```python
from build123d import *

# Parameters (mm, degrees)
BOSS_EXTRUDE1_DEPTH = 28
FILLET1_R           = 1
SWEEP1_PROFILE_R    = 0.7
LPATTERN1_COUNT     = 2
LPATTERN1_PITCH     = 2.5


with BuildPart() as part:
    # Sketch1 → Boss-Extrude1 (new body)
    with BuildSketch(Plane(origin=(0, 0, 0), x_dir=(0, 0, -1), z_dir=(1, 0, 0))):
        Polygon((0, 0), (0, 31), (2, 31), (5.7, 24), (5.7, 0), align=None)
    extrude(amount=BOSS_EXTRUDE1_DEPTH)

    # Fillet1
    fillet1_edges = [part.edges().sort_by_distance(p)[0] for p in [
        (28, 15.5, 0),
        (28, 31, -1),
        (28, 27.5, -3.85),
        (28, 12, -5.7),
        (0, 27.5, -3.85),
        (0, 31, -1),
        (0, 15.5, 0),
        (0, 0, -2.85),
        (0, 12, -5.7),
        (28, 0, -2.85),
        (14, 24, -5.7),
        (14, 31, -2),
        (14, 31, 0),
        (14, 0, 0),
        (14, 0, -5.7),
    ]]
    fillet(fillet1_edges, radius=FILLET1_R)

    # Sweep1: sweep along a path in Sketch2
    with BuildLine(Plane.XY.offset(-1.3)) as sweep1_path:
        ThreePointArc((2.353185581, 32.918653967), (1.45227767, 31.219358637), (2.297855958, 29.491864196))
    # Sweep1 profile (on start of the path) → Sweep1 (sweep)
    with BuildSketch(Plane(origin=(2.353185581, 32.918653967, -1.3), x_dir=(0.5744773116902536, -0.8185205057621582, 0), z_dir=(-0.8185205057621582, -0.5744773116902536, 0))):
        Circle(SWEEP1_PROFILE_R)
    sweep1 = sweep(path=sweep1_path.line)

    # LPattern1: Sweep1 ×2
    with Locations(*[(i * LPATTERN1_PITCH, 0, 0) for i in range(1, LPATTERN1_COUNT)]):
        add(sweep1)


solid = part.part
```
Here's how the part is built. I have some questions about the finished solid (model axes, mm). Give positions to 0.01 mm unless a question says otherwise; leave off trailing zeros. Loops run counter-clockwise (first coordinate to the right, second up) from the corner with the lowest first, then second, coordinate; pieces in that order, holes last. Notation, with made-up numbers: M 78,23.5 L 132,23.5 A28 cw 132,48.5 Z; hole C 49,88 d5. An arc over 180 degrees is marked long. Return JSON: item names as keys, results as strings.
Item 1: Imagine slicing it at A-A on x = 19.25. List the corners of the cut face in (y, z) for me.
A:
{"outline": "M 0,-4.7 A1 ccw 1,-5.7 L 23.75,-5.7 A1 ccw 24.22,-5.58 L 30.47,-2.28 A1 ccw 31,-1.4 L 31,-1 A1 ccw 30,0 L 1,0 A1 ccw 0,-1 Z"}
Item 2: Please list where these lines run through material, in increasing order: line 1 (Y direction, x = 13.75, z = -0.9); line 2 (Y direction, x = 11.75, z = -3.85); line 3 (X direction, y = 29.5, z = -0.55).
A:
{"line 1": "y = 0.01 to 30.99", "line 2": "y = 0 to 27.5", "line 3": "x = 0.11 to 27.89"}
Item 3: Thinking about a two-plate mould opening in X: for faces 1 (the cylindrical face through (0.3, 27.17, -3.7)), 2 (the flat face through (13.82, 27.39, -3.91)), 3 (the flat face through (2.348, 32.927, -1.29)), which applies, released by +X, released by -X, zero draft, split by the parting line, or undercut?
A:
{"face 1": "released by -X", "face 2": "zero draft", "face 3": "undercut"}
Item 4: I'm going to push a flat-ended pin straight in: pin 1 Ø2 at (x, z) = (17, -3) entering from +Y. Where does the tip first touch, or does it pass through?
A:
{"pin 1": "stops at y = 30.8"}
